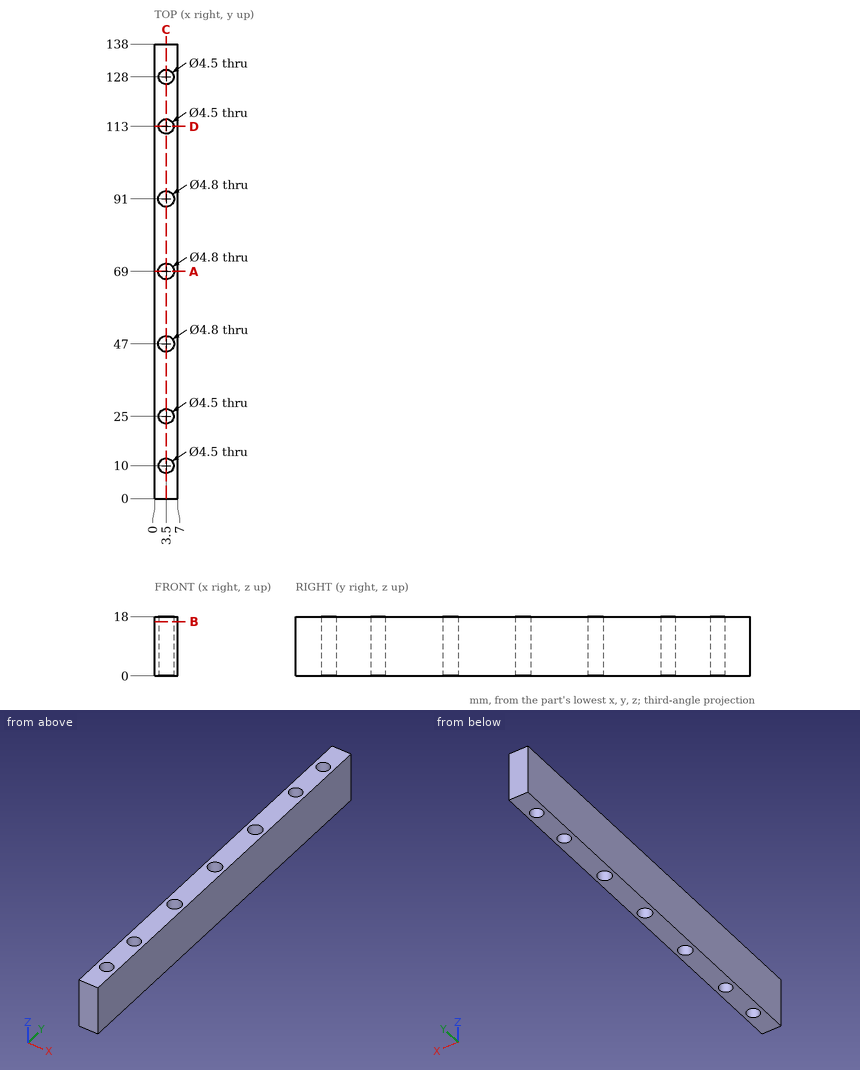
Design review of the part shown in the three views and the two pictorial views. Dimensions are in mm from the part's minimum x, y and z. Give positions to 0.01 mm unless a question says otherwise; leave off trailing zeros. Write each loop counter-clockwise with the first axis right and the second up, starting at its lowest first coordinate (ties: lowest second). Pieces come first, ordered by that corner, then holes. Notation, with made-up numbers: (33.25, 21.5) - (46.25, 21.5) arc R26 cw to (46.25, 52.5) - close; hole circle Ø10 at (37, 15). An arc over 180 degrees is marked (long way). Return JSON: item names as keys, results as strings. Group by question number.
(1) We need section D-D, the plane y = 113. Give the boundary of the cut face in (x, z).
(2) We need section C-C, the plane x = 3.5. Give the number of separate pieces and of enclosed holes in the cut face, then the cut area to 3 significant figures.
(3) We need section A-A, the plane y = 69. Give the boundary of the cut face in (x, z), then the cut area to 3 significant figures.
(4) We need section B-B, the plane z = 16.5. Give the boundary of the cut face in (x, y).
(5) To check wall thickness, follow probe 1 along X at (y, z) = (23.5, 11.25). State the ranges of the line that lie inside material, in increasing order.
(6) Insertion check: pin 1 (4 mm diameter, centred on x = 3.5, y = 69, fed in from +Z). The pin has a flat end and moves straight along its axis. Give the tip position at first contact, or say it passes through.
Reported:
{
 "1": {"outline": "(0, 0) - (1.25, 0) - (1.25, 18) - (0, 18) - close; (5.75, 0) - (7, 0) - (7, 18) - (5.75, 18) - close"},
 "2": {"separate pieces": "8", "enclosed holes": "0", "area": "1,900 mm2"},
 "3": {"outline": "(0, 0) - (1.1, 0) - (1.1, 18) - (0, 18) - close; (5.9, 0) - (7, 0) - (7, 18) - (5.9, 18) - close", "area": "39.6 mm2"},
 "4": {"outline": "(0, 0) - (7, 0) - (7, 138) - (0, 138) - close; hole circle Ø4.8 at (3.5, 47); hole circle Ø4.8 at (3.5, 69); hole circle Ø4.8 at (3.5, 91); hole circle Ø4.5 at (3.5, 10); hole circle Ø4.5 at (3.5, 25); hole circle Ø4.5 at (3.5, 113); hole circle Ø4.5 at (3.5, 128)"},
 "5": {"probe 1": "x = 0 to 1.82, 5.18 to 7"},
 "6": {"pin 1": "passes through"}
}
